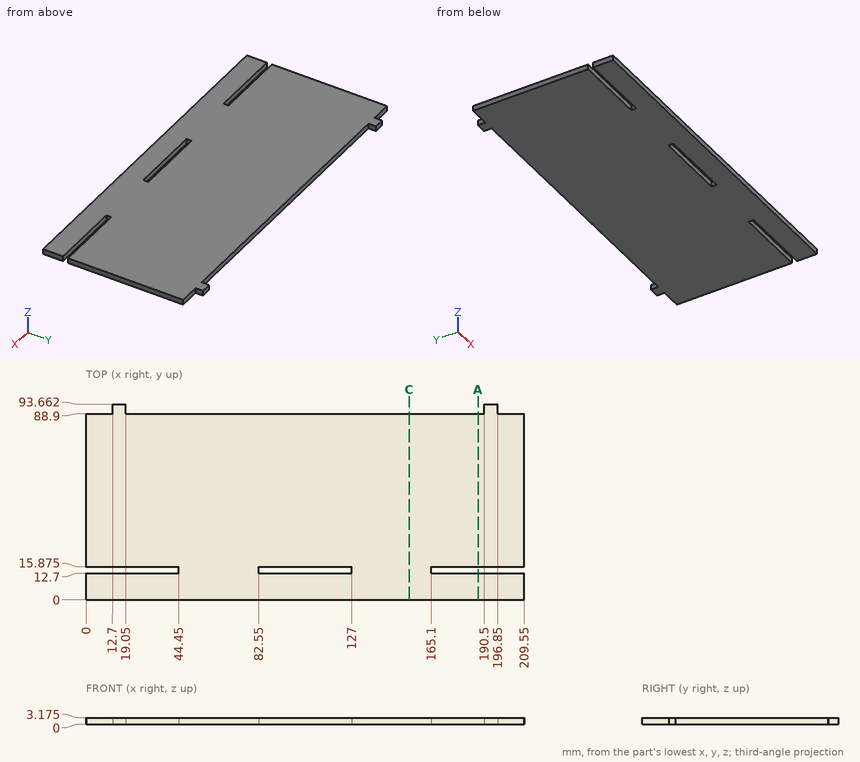
Answer from the drawing. Dimensions are ordinates in mm from the lowest x, y and z of the part. Round coordinates to 2 decimals unless told otherwise and drop trailing zeros. Order: outer loops, then holes, each group sorted by start corner. A loop starts at its lowest first (then second) coordinate and runs counter-clockwise, first axis right, second up.
1) The part is cut by section A-A on x = 187.5. Write down the section's boundary in (y, z) (1 decimal), plus the area to 3 significant figures.
2) The part is cut by section C-C on x = 154.5. Write down the section's boundary in (y, z) (1 decimal).
3) Flat-ended cylindrical pins translate along their axes: pin 1 (1.6 mm diameter, centred on y = 91.5, z = 1, fed in from +X); pin 2 (1.6 mm diameter, centred on y = 14, z = 2, fed in from -X); pin 3 (1.6 mm diameter, centred on x = 124.5, z = 1.5, fed in from +Y). Find the tip coordinate at first contact, or state that the pin passes through.
4) Straight lines are drawn through the part: L1, parallel to Y at x = 87.5, z = 0.55 (1 decimal); L2, parallel to Y at x = 141, z = 0.6; L3, parallel to X at y = 14.5, z = 0.45. For each, find the intervals that lie inside material, in ascending order.
Resolved:
1. outline: (0, 0) - (12.7, 0) - (12.7, 3.2) - (0, 3.2) - close; (15.9, 0) - (88.9, 0) - (88.9, 3.2) - (15.9, 3.2) - close
1. area: 272 mm2
2. outline: (0, 0) - (88.9, 0) - (88.9, 3.2) - (0, 3.2) - close
3. pin 1: stops at x = 196.85
3. pin 2: stops at x = 44.45
3. pin 3: stops at y = 88.9
4. L1: y = 0 to 12.7, 15.9 to 88.9
4. L2: y = 0 to 88.9
4. L3: x = 44.45 to 82.55, 127 to 165.1
